Can you work these out from the model? Positions are in its coordinate system, mm. A direction names the side the tool comes from. Coordinates: 2 decimals unless noted, no trailing zeros. Loops run counter-clockwise (first coordinate to the right, second up) from the corner with the lowest first, then second, coordinate; pieces in that order, holes last.
```python
from build123d import *

# Parameters (mm, degrees)
F0_W        = 100.18889606
F0_H        = 74.0776211023
F1_DEPTH    = 127
F2_W        = 51.0549172759
F2_H        = 49.9856282473
F3_DEPTH    = 76.2
F4_T1_DEPTH = 305.0222773169
F4_T3_DEPTH = 303.9856282473
F6_D        = 6.35


# Not quite as in the source:
# - a fillet or chamfer that OpenCascade refuses, or shapes differently, is made with other operations: its cross-section is extruded or revolved along the edge and cut away or added


with BuildPart() as f1:
    # F0 (on Front) → F1 (new body)
    with BuildSketch(Plane.XZ):
        with Locations((50.09444803, 37.0388105512)):
            Rectangle(F0_W, F0_H)
    extrude(amount=F1_DEPTH)

    # F2 (on face) → F3 (join)
    with BuildSketch(Plane.XY.offset(74.0776211023)):
        with Locations((74.661437422, -102.0071858764)):
            Rectangle(F2_W, F2_H)
    extrude(amount=F3_DEPTH)

    # F4: fillet of radius 50.8 on 2 edges, made by hand

    # F4_s2 → F4_t1 (cut)
    with BuildSketch(Plane.YZ.offset(-77.8497012364)):
        with BuildLine():
            ThreePointArc((-77.0143717527, 99.4841490941), (-91.6065681392, 135.1160864184), (-127, 150.2776211023))
            Line((-127, 150.2776211023), (-77.0143717527, 150.2776211023))
            Line((-77.0143717527, 150.2776211023), (-77.0143717527, 99.4841490941))
        make_face()
    extrude(amount=F4_T1_DEPTH, mode=Mode.SUBTRACT)

    # F4_s4 → F4_t3 (cut)
    with BuildSketch(Plane.XZ.offset(-49.9856282473)):
        with BuildLine():
            ThreePointArc((49.1339787841, 99.4776211023), (64.0129542998, 135.3986455866), (99.9339787841, 150.2776211023))
            Line((99.9339787841, 150.2776211023), (49.1339787841, 150.2776211023))
            Line((49.1339787841, 150.2776211023), (49.1339787841, 99.4776211023))
        make_face()
    extrude(amount=F4_T3_DEPTH, mode=Mode.SUBTRACT)

    # F6 (through all)
    with Locations(Plane(origin=(0, 0, 0), x_dir=(-1, 0, 0), z_dir=(0, 1, 0))):
        with Locations((-53.5700023174, 41.735380888)):
            Hole(F6_D / 2)


solid = f1.part
```
Item 1: Suppose I cut it at A-A, the plane y = -90.5. Please give me the cut outline in (x, z) (3 decimals).
Results are:
outline: (0, 0) - (100.189, 0) - (100.189, 133.956) - (62.626, 133.956) arc R50.8 ccw to (49.134, 99.478) - (49.134, 74.078) - (0, 74.078) - close; hole circle Ø6.35 at (53.57, 41.735)
Item 2: On a 3-axis mill with a long thin cutter (end or side, diameter ignored), from which of +Z, -Z, +X, -X, +Y, -Y can I reach the whole of each face in a straight line? I mean faces 5 (the face through (74, -77.014, 87)), 6 (the face through (49.134, -102, 87)), 7 (the face through (49, 0, 38)). Say none if no direction works.
Results are:
face 5: +Z, +X, -X, +Y
face 6: +Z, -X, +Y, -Y
face 7: +Z, -Z, +X, -X, +Y
Item 3: I'm going to push flat-ended pins straight in: P1, Ø20.5, axis at x = 79.5, z = 87, coming from the +Y side; P2, Ø20.5, axis at y = -108, z = 91, coming from the -X side; P3, Ø2, axis at x = 68, z = 114, coming from the +Y side. Where does each tip first touch, or does it pass through?
Results are:
P1: stops at y = -77.01
P2: stops at x = 49.13
P3: stops at y = -78.85
Item 4: Suppose I cut it at C-C, the plane z = 82.5. Please give me the cut outline in (x, y), plus the area to 3 significant figures.
Results are:
outline: (49.13, -127) - (100.19, -127) - (100.19, -77.01) - (49.13, -77.01) - close
area: 2,550 mm2
Item 5: Suppose I cut it at D-D, the plane x = 64.5. Please give me the cut outline in (y, z).
Results are:
outline: (-127, 0) - (0, 0) - (0, 74.08) - (-77.01, 74.08) - (-77.01, 99.48) arc R50.8 ccw to (-92.37, 135.88) - (-127, 135.88) - close
Item 6: We'd pull the mould along X, two halves only. Please class faces 1 (the face through (49, -63, 0)), 2 (the face through (100.189, -79, 57)), 3 (the face through (0, -63, 37)), 4 (the face through (55.3, -64.4, 44.4)): +X half, -X half, draft (parallel to the pull), parting line (faces both ways), or undercut.
Results are:
face 1: draft
face 2: +X half
face 3: -X half
face 4: undercut
Item 7: I need wall thicknesses on line 1 along Z through (x, y) = (87, -74.5); line 2 along X through (y, z) = (-99, 44); line 3 along Y through (x, z) = (93, 93). Which ranges of each line are inside material? Lowest first, please.
Results are:
line 1: z = 0 to 74.08
line 2: x = 0 to 51.34, 55.8 to 100.19
line 3: y = -127 to -77.01
Item 8: Suppose I cut it at B-B, the plane x = 53. Please give me the cut outline in (y, z), plus the area to 3 significant figures.
Results are:
outline: (-127, 0) - (0, 0) - (0, 38.61) - (-127, 38.61) - close; (-127, 44.86) - (0, 44.86) - (0, 74.08) - (-77.01, 74.08) - (-77.01, 99.48) arc R50.8 ccw to (-80.88, 118.92) - (-127, 118.92) - close
area: 10,800 mm2
